Geometry: final body of the model. Coordinates: model frame, mm. Face numbers are marked on the shaded views. Give positions to 0.01 mm unless a question says otherwise; leave off trailing zeros. Write each loop counter-clockwise with the first axis right and the second up, starting at its lowest first coordinate (ties: lowest second). Pieces come first, ordered by that corner, then holes.
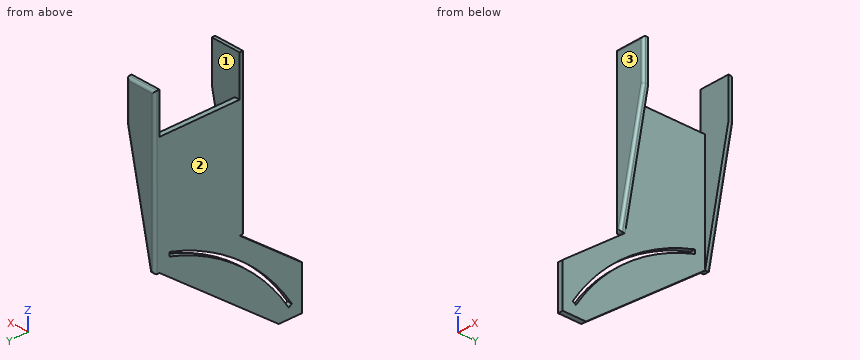
```python
from build123d import *

# Parameters (mm, degrees)
BOSS_EXTRUDE1_DEPTH = 3.175
BOSS_EXTRUDE2_DEPTH = 3.175
FILLET1_R           = 1.5875
BOSS_EXTRUDE3_DEPTH = 3.175
FILLET2_R           = 1.5875


with BuildPart() as part:
    # Sketch1 → Boss-Extrude1 (new body)
    with BuildSketch(Plane(origin=(0, 0, 0), x_dir=(0, 0, -1), z_dir=(1, 0, 0))):
        Polygon((-120.564627305, -30.226), (-63.414627305, -105.80178633), (-63.414627305, -120.523753631), (-90.752572968, -120.523753631), (-120.620560185, -81.026), (-193.675, -81.026), (-193.675, -30.226), align=None)
        with BuildLine():
            Line((-129.390973316, -36.576), (-126.914627305, -36.576))
            ThreePointArc((-126.914627305, -36.576), (-105.349927235, -79.665043976), (-69.764627305, -112.15178633))
            Line((-69.764627305, -112.15178633), (-71.022403038, -114.173753631))
            ThreePointArc((-71.022403038, -114.173753631), (-107.455726685, -80.827560609), (-129.390973316, -36.576))
        make_face(mode=Mode.SUBTRACT)
    extrude(amount=BOSS_EXTRUDE1_DEPTH)

    # Sketch2 → Boss-Extrude2 (add)
    with BuildSketch(Plane(origin=(0, -30.226, 0), x_dir=(1, 0, 0), z_dir=(0, 1, 0))):
        Polygon((0, -120.564627305), (3.175, -120.564627305), (19.05, -193.675), (19.05, -219.075), (0, -219.075), align=None)
    extrude(amount=BOSS_EXTRUDE2_DEPTH)

    # Fillet1
    # the kernel refuses this fillet: 1.5875 mm, written as the material it adds along each edge
    with BuildSketch(Plane(origin=(0, -30.226, 120.564627305), x_dir=(0, -0.7976221020191943, -0.6031575104153825), z_dir=(1, 0, 0))) as fillet1_piece_1:
        with BuildLine():
            CenterArc((FILLET1_R * 0.335530760185, FILLET1_R), FILLET1_R, 232.903626037, 37.096373963)
            Line((-FILLET1_R * 0.267626750231, FILLET1_R * 0.202377897981), (0, 0))
            Line((0, 0), (FILLET1_R * 0.335530760185, 0))
        make_face()
    extrude(amount=3.175)
    # the kernel refuses this fillet: 1.5875 mm, written as the material it takes off along each edge
    with BuildSketch(Plane(origin=(0, -27.051, 223.04375), x_dir=(0, -1, 0), z_dir=(0, 0, -1))) as fillet1_2_piece_1:
        with BuildLine():
            CenterArc((FILLET1_R, -FILLET1_R), FILLET1_R, 90, 90)
            Line((0, -FILLET1_R), (0, 0))
            Line((0, 0), (FILLET1_R, 0))
        make_face()
    extrude(amount=106.447872695, mode=Mode.SUBTRACT)
    with BuildSketch(Plane(origin=(23.01875, -27.051, 219.075), x_dir=(0, -1, 0), z_dir=(-1, 0, 0))) as fillet1_2_piece_2:
        with BuildLine():
            CenterArc((FILLET1_R, -FILLET1_R), FILLET1_R, 90, 90)
            Line((0, -FILLET1_R), (0, 0))
            Line((0, 0), (FILLET1_R, 0))
        make_face()
    extrude(amount=26.9875, mode=Mode.SUBTRACT)
    with BuildSketch(Plane(origin=(19.05, -27.051, 189.70625), x_dir=(-1, 0, 0), z_dir=(0, 0, 1))) as fillet1_2_piece_3:
        with BuildLine():
            CenterArc((FILLET1_R, FILLET1_R), FILLET1_R, 180, 90)
            Line((0, FILLET1_R), (0, 0))
            Line((0, 0), (FILLET1_R, 0))
        make_face()
    extrude(amount=33.3375, mode=Mode.SUBTRACT)
    with BuildSketch(Plane(origin=(2.332859982, -27.051, 116.686254354), x_dir=(-0.9772278303307078, 0, 0.21219276054365557), z_dir=(0.21219276054365557, 0, 0.9772278303307079))) as fillet1_2_piece_4:
        with BuildLine():
            CenterArc((FILLET1_R, FILLET1_R), FILLET1_R, 180, 90)
            Line((0, FILLET1_R), (0, 0))
            Line((0, 0), (FILLET1_R, 0))
        make_face()
    extrude(amount=82.751550957, mode=Mode.SUBTRACT)
    with BuildSketch(Plane(origin=(-3.96875, -27.051, 120.564627305), x_dir=(0, 0, 1), z_dir=(1, 0, 0))) as fillet1_2_piece_5:
        with BuildLine():
            CenterArc((FILLET1_R, FILLET1_R), FILLET1_R, 180, 90)
            Line((0, FILLET1_R), (0, 0))
            Line((0, 0), (FILLET1_R, 0))
        make_face()
    extrude(amount=11.1125, mode=Mode.SUBTRACT)

    # Sketch4 → Boss-Extrude3 (add)
    with BuildSketch(Plane.XZ.offset(81.026)):
        Polygon((0, 120.620560185), (3.175, 120.620560185), (19.05, 193.675), (19.05, 219.075), (0, 219.075), align=None)
    extrude(amount=BOSS_EXTRUDE3_DEPTH)

    # Fillet2
    fillet2_edges = [part.edges().sort_by_distance(p)[0] for p in [
        (0, -84.201, 169.847780093),
        (1.5875, -84.201, 120.620560185),
        (11.1125, -84.201, 157.147780093),
        (19.05, -84.201, 206.375),
        (9.525, -84.201, 219.075),
    ]]
    fillet(fillet2_edges, radius=FILLET2_R)


solid = part.part
```
Item 1: Line query: L1, parallel to Y at x = 15.75, z = 207.5; L2, parallel to X at y = -90, z = 93 (3 decimals); L3, parallel to Y at x = 3, z = 179.5. Output: solid intervals per line, ascending.
Found:
L1: y = -84.2 to -81.03, -30.23 to -27.05
L2: x = 0 to 3.175
L3: y = -84.2 to -27.05
Item 2: Pull-direction query (Y, two-part tool) for the marked faces 1, 2 and 3; classes: +Y half, -Y half, draft (parallel to the pull), parting line (faces both ways), or undercut.
Found:
face 1: undercut
face 2: draft
face 3: -Y half
Item 3: Pin query (flat end, axial travel): pin 1 Ø8 at (y, z) = (-71.5, 180) entering from +X (3 decimals); pin 2 Ø3 at (y, z) = (-72.5, 130.5) entering from -X; pin 3 Ø1 at (x, y) = (3, -74) entering from +Z (3 decimals); pin 4 Ø1.3 at (x, y) = (1.5, -82) entering from -Z. Return the tip coordinate at first contact, or that it passes through.
Found:
pin 1: stops at x = 3.175
pin 2: stops at x = 0
pin 3: stops at z = 193.675
pin 4: stops at z = 80.92
Item 4: Section B-B, the plane z = 73.5. Return the cut outline in (x, y) (3 decimals), plus the area to 3 significant figures.
Found:
outline: (0, -120.524) - (3.175, -120.524) - (3.175, -112.595) - (0, -112.595) - close; (0, -109.74) - (3.175, -109.74) - (3.175, -92.465) - (0, -92.465) - close
area: 80.0 mm2
Item 5: Section A-A, the plane y = -98. Return the cut outline in (x, z) (3 decimals).
Found:
outline: (0, 69.314) - (3.175, 69.314) - (3.175, 88.55) - (0, 88.55) - close; (0, 92.064) - (3.175, 92.064) - (3.175, 107.785) - (0, 107.785) - close
